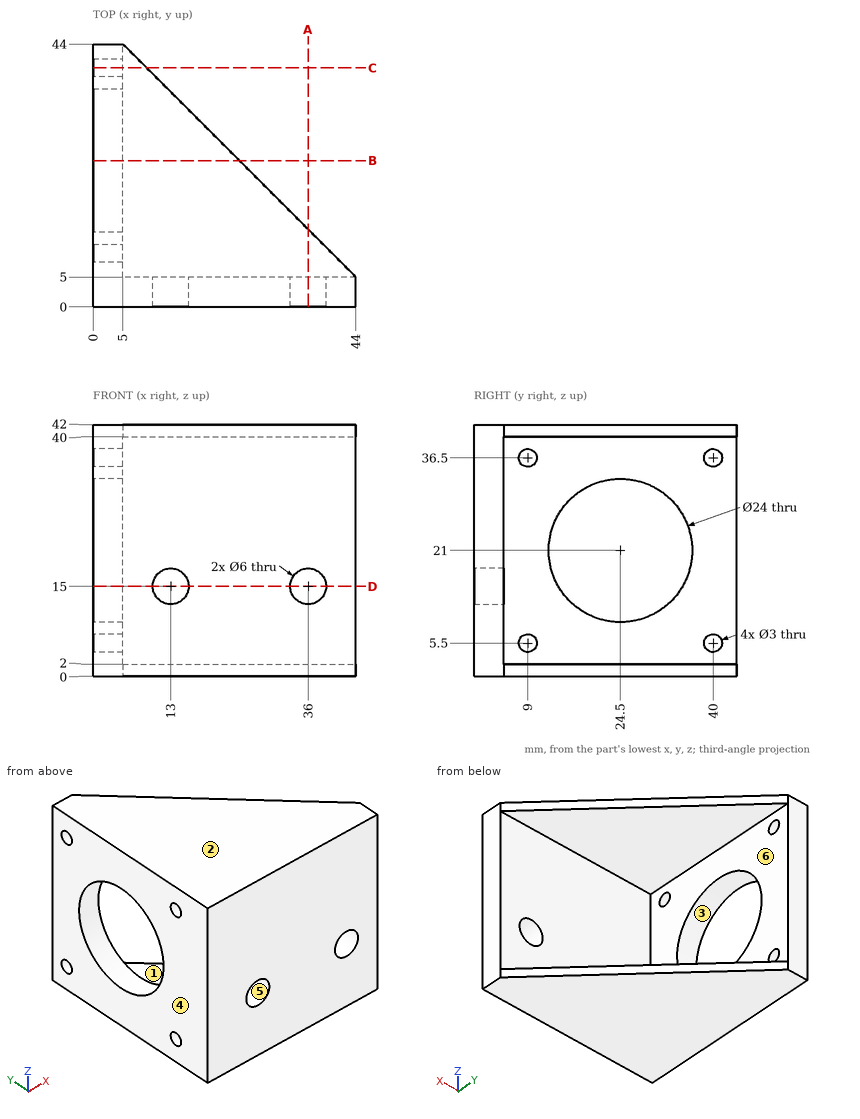
Geometry: see drawing. Coordinates: mm, zero at the bounding-box minimum. A direction names the side the tool comes from. Coordinates: 2 decimals unless noted, no trailing zeros. Write each loop counter-clockwise with the first axis right and the second up, starting at its lowest first coordinate (ties: lowest second). Pieces come first, ordered by that corner, then holes. Notation, with made-up numbers: M -22.5,14 L 6.5,14 A24 cw 6.5,36 Z; hole C -33.5,56 d6. An arc over 180 degrees is marked long. Answer as a JSON object with one key per item and string values.
1. Cut plane D-D on z = 15. Output: boundary loops of the cut face in (x, y), plus the area to 3 significant figures.
Evaluation:
{"outline": "M 0,0 L 10,0 L 10,5 L 5,5 L 5,14.11 L 0,14.11 Z; M 0,34.89 L 5,34.89 L 5,44 L 0,44 Z; M 16,0 L 33,0 L 33,5 L 16,5 Z; M 39,0 L 44,0 L 44,5 L 39,5 Z", "area": "251 mm^2"}
2. Cut plane A-A on x = 36. Output: boundary loops of the cut face in (y, z).
Evaluation:
{"outline": "M 0,0 L 13,0 L 13,2 L 5,2 L 5,12 L 0,12 Z; M 0,18 L 5,18 L 5,40 L 13,40 L 13,42 L 0,42 Z"}
3. Ray query, L1, parallel to Z at x = 2.25, y = 40; L2, parallel to Z at x = 15, y = 11.5; L3, parallel to Y at x = 38.5, z = 26.5. Return the intervals inside material, ascending.
Evaluation:
{"L1": "0 to 4, 7 to 35, 38 to 42", "L2": "0 to 2, 40 to 42", "L3": "0 to 5"}
4. Cut plane B-B on y = 24.5. Output: boundary loops of the cut face in (x, z), plus the area to 3 significant figures.
Evaluation:
{"outline": "M 0,0 L 24.5,0 L 24.5,2 L 5,2 L 5,9 L 0,9 Z; M 0,33 L 5,33 L 5,40 L 24.5,40 L 24.5,42 L 0,42 Z", "area": "168 mm^2"}
5. Access query for the marked faces 1 and 2. Directions: +Z, -Z, +X, -X, +Y, -Y. A direction counts if a zero-diameter tool reaches every point of the face in a straight line with its end or side. Return the directions, or none.
Evaluation:
{"face 1": "+X, +Y", "face 2": "+Z, +X, -X, +Y, -Y"}
6. Draft query along X for the marked faces 3, 4, 5 and 6. Return one class per face: released by +X, released by -X, zero draft, split by the parting line, or undercut.
Evaluation:
{"face 3": "zero draft", "face 4": "released by -X", "face 5": "undercut", "face 6": "released by +X"}
7. Contact query for flat-ended pins moving along their axis: P1, Ø3.5, axis at y = 9, z = 5.5, coming from the +X side; P2, Ø6, axis at x = 18.5, z = 30, coming from the +Y side. Output: stop coordinate, or through.
Evaluation:
{"P1": "x = 5", "P2": "y = 5"}
8. Cut plane C-C on y = 40. Output: boundary loops of the cut face in (x, z), plus the area to 3 significant figures.
Evaluation:
{"outline": "M 0,0 L 9,0 L 9,2 L 5,2 L 5,4 L 0,4 Z; M 0,7 L 5,7 L 5,35 L 0,35 Z; M 0,38 L 5,38 L 5,40 L 9,40 L 9,42 L 0,42 Z", "area": "196 mm^2"}
